from build123d import *

# Parameters (mm, degrees)
EXTRUDE_1_DEPTH     = 50
CUT_EXTRUDE_1_DEPTH = 73.083285164
EXTRUDE_START       = -15
EXTRUDE_2_DEPTH     = 15
SKETCH_4_3_R        = 16
SKETCH_4_3_R_2      = 9
EXTRUDE_3_DEPTH     = 18
EXTRUDE_4_DEPTH     = 15
EXTRUDE_START_2     = -45
EXTRUDE_5_DEPTH     = 45
CUT_EXTRUDE_2_DEPTH = 81.274528962


with BuildPart() as part:
    # Sketch 1 → Extrude 1 (new body)
    with BuildSketch(Plane.XY):
        with BuildLine():
            Line((-50, 0), (-18, 0))
            ThreePointArc((-18, 0), (0, 18), (18, 0))
            Line((18, 0), (50, 0))
            Line((50, 0), (50, 14))
            Line((50, 14), (19.49358869, 14))
            ThreePointArc((19.49358869, 14), (0, 24), (-19.49358869, 14))
            Line((-19.49358869, 14), (-50, 14))
            Line((-50, 14), (-50, 0))
        make_face()
    extrude(amount=-EXTRUDE_1_DEPTH)

    # Sketch 2 → Cut-Extrude 1 (cut, through all)
    with BuildSketch(Plane(origin=(0, 14, 0), x_dir=(1, 0, 0), z_dir=(0, 1, 0))):
        with BuildLine():
            Line((-62, 33), (-38, 33))
            ThreePointArc((-38, 33), (-30, 25), (-38, 17))
            Line((-38, 17), (-62, 17))
            ThreePointArc((-62, 17), (-70, 25), (-62, 33))
        make_face()
        with BuildLine():
            Line((62, 33), (38, 33))
            ThreePointArc((38, 33), (30, 25), (38, 17))
            Line((38, 17), (62, 17))
            ThreePointArc((62, 17), (70, 25), (62, 33))
        make_face()
    extrude(amount=-CUT_EXTRUDE_1_DEPTH, mode=Mode.SUBTRACT)

    # Sketch 4 → Extrude 2 (add)
    with BuildSketch(Plane(origin=(0, 0, -50), x_dir=(-1, 0, 0), z_dir=(0, 0, -1)).offset(EXTRUDE_START)):
        with BuildLine():
            ThreePointArc((-19.49358869, 14), (0, 24), (19.49358869, 14))
            Line((19.49358869, 14), (17.69427427, 38))
            Line((17.69427427, 38), (-17.69427427, 38))
            Line((-17.69427427, 38), (-19.49358869, 14))
        make_face()
    extrude(amount=EXTRUDE_2_DEPTH)



with BuildPart() as body_2:
    # Sketch 4_3 → Extrude 3 (new body)
    with BuildSketch(Plane(origin=(0, 0, -50), x_dir=(-1, 0, 0), z_dir=(0, 0, -1))):
        with Locations((0, 60)):
            Circle(SKETCH_4_3_R)
        with Locations((0, 60)):
            Circle(SKETCH_4_3_R_2, mode=Mode.SUBTRACT)
    extrude(amount=-EXTRUDE_3_DEPTH)


with BuildPart() as part_1:
    add(part.part)

    add(body_2.part)  # Extrude 4 merges body 2
    # Sketch 4_4 → Extrude 4 (add)
    with BuildSketch(Plane(origin=(0, 0, -50), x_dir=(-1, 0, 0), z_dir=(0, 0, -1))):
        with BuildLine():
            Line((0, 44), (0, 38))
            Line((0, 38), (17.69427427, 38))
            Line((17.69427427, 38), (15.955222944, 61.196185946))
            ThreePointArc((15.955222944, 61.196185946), (15.988801817, 60.598511863), (16, 60))
            ThreePointArc((16, 60), (11.313708499, 48.686291501), (0, 44))
        make_face()
        with BuildLine():
            Line((-17.69427427, 38), (0, 38))
            Line((0, 38), (0, 44))
            ThreePointArc((0, 44), (-11.729001985, 49.117421609), (-15.955222944, 61.196185946))
            Line((-15.955222944, 61.196185946), (-17.69427427, 38))
        make_face()
    extrude(amount=-EXTRUDE_4_DEPTH)

    # Sketch 4_5 → Extrude 5 (add)
    with BuildSketch(Plane(origin=(0, 0, -50), x_dir=(-1, 0, 0), z_dir=(0, 0, -1)).offset(EXTRUDE_START_2)):
        with BuildLine():
            Line((0, 38), (0, 24))
            ThreePointArc((0, 24), (10.95445115, 21.354156504), (19.49358869, 14))
            Line((19.49358869, 14), (17.69427427, 38))
            Line((17.69427427, 38), (0, 38))
        make_face()
        with BuildLine():
            ThreePointArc((-19.49358869, 14), (-10.95445115, 21.354156504), (0, 24))
            Line((0, 24), (0, 38))
            Line((0, 38), (-17.69427427, 38))
            Line((-17.69427427, 38), (-19.49358869, 14))
        make_face()
    extrude(amount=EXTRUDE_5_DEPTH)

    # Sketch 5 → Cut-Extrude 2 (cut, through all)
    with BuildSketch(Plane(origin=(0, 38, 0), x_dir=(1, 0, 0), z_dir=(0, 1, 0))):
        with BuildLine():
            ThreePointArc((6, 20), (5.632962232, 22.066334072), (4.576754501, 23.879860596))
            Line((4.576754501, 23.879860596), (-4.576754501, 16.120139404))
            ThreePointArc((-4.576754501, 16.120139404), (2.066334072, 14.367037768), (6, 20))
        make_face()
        with BuildLine():
            Line((-4.576754501, 16.120139404), (4.576754501, 23.879860596))
            ThreePointArc((4.576754501, 23.879860596), (-3.879860596, 24.576754501), (-4.576754501, 16.120139404))
        make_face()
    extrude(amount=-CUT_EXTRUDE_2_DEPTH, mode=Mode.SUBTRACT)


solid = part_1.part
Work out the finished part from the listing and answer in its coordinate system (mm). A direction names the side the tool comes from. Coordinates: 2 decimals unless noted, no trailing zeros. Write each loop counter-clockwise with the first axis right and the second up, starting at its lowest first coordinate (ties: lowest second). Pieces come first, ordered by that corner, then holes. Notation, with made-up numbers: (22.25, -7.5) - (49.25, -7.5) arc R19 cw to (49.25, 23.5) - close; hole circle Ø7 at (13, 56.25). An arc over 180 degrees is marked (long way). One line per question, with ' | ' between items.
1) Find section A-A, the plane z = -12.5. Determine the outline of the cut face in (x, y).
Checks:
outline: (-50, 0) - (-18, 0) arc R18 cw to (18, 0) - (50, 0) - (50, 14) - (19.49, 14) - (17.69, 38) - (-17.69, 38) - (-19.49, 14) - (-50, 14) - close
2) Flat-ended cylindrical pins translate along their axes: P1, Ø9.5, axis at x = -45, y = 5, coming from the +Z side; P2, Ø2, axis at x = 17.5, y = 22.5, coming from the +Z side; P3, Ø15.5, axis at x = 0, z = -20, coming from the +Y side; P4, Ø8, axis at y = 20, z = -44.5, coming from the -X side. Find the tip coordinate at first contact, or state that the pin passes through.
Checks:
P1: z = 0 | P2: z = -5 | P3: y = 38 | P4: x = -19.34
3) Find section B-B, the plane x = 0. Determine the outline of the cut face in (y, z), and give its area (3 significant figures).
Checks:
outline: (18, -50) - (51, -50) - (51, -32) - (44, -32) - (44, -35) - (38, -35) - (38, -26) - (18, -26) - close; (18, -14) - (38, -14) - (38, -5) - (24, -5) - (24, 0) - (18, 0) - close; (69, -50) - (76, -50) - (76, -32) - (69, -32) - close | area: 1,030 mm2
4) For faces 4 (the face through (0, 38, -13)), 5 (the face through (-28, 14, -25)), 6 (the face through (28, 14, -25)), 7 (the face through (0, 24, -2)), 8 (the face through (-7, 53, -32)), determine the directions among +Z, -Z, +X, -X, +Y, -Y from which every point of the face is accessible in a straight line to the end or side of a thin tool.
Checks:
face 4: +Z, +X, -X | face 5: +Z, -Z, -X, +Y | face 6: +Z, -Z, +X, +Y | face 7: +Z, +Y | face 8: +Z, +X, -X, +Y
5) Find section C-C, the plane y = 60. Determine the outline of the cut face in (x, z).
Checks:
outline: (-16.04, -50) - (-9, -50) - (-9, -32) - (-16, -32) - (-16, -35) - (-16.04, -35) - close; (9, -50) - (16.04, -50) - (16.04, -35) - (16, -35) - (16, -32) - (9, -32) - close
6) Find section D-D, the plane z = -41. Determine the outline of the cut face in (x, y).
Checks:
outline: (-50, 0) - (-18, 0) arc R18 cw to (18, 0) - (50, 0) - (50, 14) - (19.49, 14) - (15.96, 61.2) arc R16 ccw to (-15.96, 61.2) - (-19.49, 14) - (-50, 14) - close; hole circle Ø18 at (0, 60)
7) The mould has two halves that part along Y. Classify faces 1 (the face through (-44, 7, -17)), 2 (the face through (27, 0, -25)), 3 (the face through (0, 42, -35)): +Y half, -Y half, draft (parallel to the pull), parting line (faces both ways), or undercut.
Checks:
face 1: draft | face 2: -Y half | face 3: undercut
8) Consider probe 1 along Y at (x, z) = (0, -41); probe 2 along Y at (x, z) = (31, -14); probe 3 along X at (y, z) = (56, -39). Determine where each line is inside the solid, lowest interval first. Write a range as [from, to].
Checks:
probe 1: [18, 51], [69, 76] | probe 2: [0, 14] | probe 3: [-16.34, -8.06], [8.06, 16.34]
